```python
from build123d import *

# Parameters (mm, degrees)
SKETCH1_R           = 23.925
SKETCH1_R_2         = 5
BOSS_EXTRUDE1_DEPTH = 5.5
SKETCH2_R           = 17.5
SKETCH2_R_2         = 4
BOSS_EXTRUDE3_DEPTH = 14
CUT_EXTRUDE1_DEPTH  = 11
CIRPATTERN10_COUNT  = 30
SKETCH4_R           = 27
SKETCH4_R_2         = 21
BOSS_EXTRUDE4_DEPTH = 1
BOSS_EXTRUDE5_START = 1
SKETCH5_R           = 27
SKETCH5_R_2         = 21
BOSS_EXTRUDE5_DEPTH = 1


with BuildPart() as part:
    # Sketch1 → Boss-Extrude1 (new, symmetric)
    with BuildSketch(Plane(origin=(0, 0, 0), x_dir=(1, 0, 0), z_dir=(0, 1, 0))):
        with Locations(Location((0, 0, 0), (0, 0, 270))):
            Circle(SKETCH1_R)
        with Locations(Location((0, 0, 0), (0, 0, 270))):
            Circle(SKETCH1_R_2, mode=Mode.SUBTRACT)
    extrude(amount=BOSS_EXTRUDE1_DEPTH, both=True)

    # Sketch2 → Boss-Extrude3 (add)
    with BuildSketch(Plane.XZ.offset(5.5)):
        with Locations(Location((0, 0, 0), (0, 0, 270))):
            Circle(SKETCH2_R)
        with Locations(Location((0, 0, 0), (0, 0, 270))):
            Circle(SKETCH2_R_2, mode=Mode.SUBTRACT)
    extrude(amount=BOSS_EXTRUDE3_DEPTH)

    # Sketch3 → Cut-Extrude1 (cut)
    with BuildSketch(Plane(origin=(0, 5.5, 0), x_dir=(1, 0, 0), z_dir=(0, 1, 0))):
        Polygon((-1, 21.84125888), (1, 21.84125888), (2, 23.84125888), (2.094207699, 23.965937646), (-2.062339383, 23.965937646), (-2, 23.84125888), align=None)
    cut_extrude1 = extrude(amount=-CUT_EXTRUDE1_DEPTH, mode=Mode.SUBTRACT)

    # CirPattern10: Cut-Extrude1 ×30 about axis
    cirpattern10_axis = Axis((0, 0, 0), (0, 1, 0))
    for i in range(1, CIRPATTERN10_COUNT):
        add(cut_extrude1.rotate(cirpattern10_axis, i * 360 / CIRPATTERN10_COUNT), mode=Mode.SUBTRACT)

    # Sketch4 → Boss-Extrude4 (add)
    with BuildSketch(Plane(origin=(0, 5.5, 0), x_dir=(1, 0, 0), z_dir=(0, 1, 0))):
        with Locations(Location((0, 0, 0), (0, 0, 270))):
            Circle(SKETCH4_R)
        with Locations(Location((0, 0, 0), (0, 0, 270))):
            Circle(SKETCH4_R_2, mode=Mode.SUBTRACT)
    extrude(amount=BOSS_EXTRUDE4_DEPTH)

    # Sketch5 → Boss-Extrude5 (add)
    with BuildSketch(Plane.XZ.offset(5.5).offset(BOSS_EXTRUDE5_START)):
        with Locations(Location((0, 0, 0), (0, 0, 90))):
            Circle(SKETCH5_R)
        with Locations(Location((0, 0, 0), (0, 0, 90))):
            Circle(SKETCH5_R_2, mode=Mode.SUBTRACT)
    extrude(amount=-BOSS_EXTRUDE5_DEPTH)


solid = part.part
```
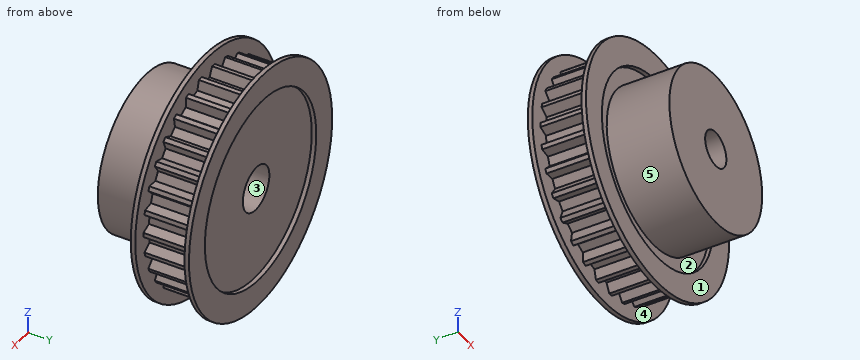
Here's how the part is built. I have some questions about the finished solid (model axes, mm). Face numbers are marked on the shaded views. A direction names the side the tool comes from. Round coordinates to 2 decimals unless told otherwise and drop trailing zeros. Loops run counter-clockwise (first coordinate to the right, second up) from the corner with the lowest first, then second, coordinate; pieces in that order, holes last.
1. Suppose I cut it at C-C, the plane z = 7. Please give me the cut outline in (x, y), and give its area (3 significant figures).
Answers:
outline: (-26.08, -6.5) - (-19.8, -6.5) - (-19.8, -5.5) - (-16.04, -5.5) - (-16.04, -19.5) - (16.04, -19.5) - (16.04, -5.5) - (19.8, -5.5) - (19.8, -6.5) - (26.08, -6.5) - (26.08, -5.5) - (20.69, -5.5) - (20.69, 5.5) - (26.08, 5.5) - (26.08, 6.5) - (19.8, 6.5) - (19.8, 5.5) - (-19.8, 5.5) - (-19.8, 6.5) - (-26.08, 6.5) - (-26.08, 5.5) - (-20.69, 5.5) - (-20.69, -5.5) - (-26.08, -5.5) - close
area: 929 mm2
2. For the marked faces 3, 4 and 5, which set-ups out of +Z, -Z, +X, -X, +Y, -Y let a thin tool reach every point of the face, with its end or its side?
Answers:
face 3: +Y
face 4: none
face 5: -Y
3. Suppose I cut it at B-B, the plane y = -8.25. Please give me the cut outline in (x, z), and give its area (3 significant figures).
Answers:
outline: circle Ø35 at (0, 0); hole circle Ø8 at (0, 0)
area: 912 mm2
4. Will these pins go through, and if not, where does the flat tip stop? pin 1 (10 mm diameter, centred on x = 7.5, y = 3.5, fed in from +Z); pin 2 (6 mm diameter, centred on x = 14, z = 0, fed in from +Y); pin 3 (1.6 mm diameter, centred on x = 0, y = -1.5, fed in from -Z).
Answers:
pin 1: stops at z = 26.84
pin 2: stops at y = 5.5
pin 3: stops at z = -21.84
5. Thinking about a two-plate mould opening in Z: for the marked faces 1 and 2, which applies, released by +Z, released by -Z, zero draft, split by the parting line, or undercut?
Answers:
face 1: zero draft
face 2: undercut
6. If I drill on probe 1 along X at (y, z) = (-6.2, 0); probe 2 along Y at (x, z) = (24.5, -8.5); probe 3 along X at (y, z) = (-14.25, 0), over which ranges is the centre line in solid material (lowest first)?
Answers:
probe 1: x = -27 to -21, -17.5 to -4, 4 to 17.5, 21 to 27
probe 2: y = -6.5 to -5.5, 5.5 to 6.5
probe 3: x = -17.5 to -4, 4 to 17.5
